Design review of the part built by this model. Coordinates are the model's own, in mm. A direction names the side the tool comes from. Coordinates: 2 decimals unless noted, no trailing zeros. Loops run counter-clockwise (first coordinate to the right, second up) from the corner with the lowest first, then second, coordinate; pieces in that order, holes last. Notation, with made-up numbers: (-5.75, 24) - (46.25, 24) arc R23 ccw to (46.25, 34) - close; hole circle Ø7 at (54.25, 34). An arc over 180 degrees is marked (long way). One line per question, with ' | ' between items.
from build123d import *

# Parameters (mm, degrees)
F0_W           = 150
F0_H           = 150
F0_R           = 30
F1_DEPTH       = 50
F2_R           = 37.5
F2_R_2         = 30
F3_DEPTH       = 40
F4_R           = 41.25
F4_R_2         = 37.5
F5_DEPTH       = 7
F7_D           = 10.2
F7_DEPTH       = 40
F7_CSINK_D     = 12
F7_CSINK_ANGLE = 90
F7_TIP         = 3.064389157
F8_R           = 15


with BuildPart() as f1:
    # F0 (on Top) → F1 (new body)
    with BuildSketch(Plane.XY):
        Rectangle(F0_W, F0_H)
        Circle(F0_R, mode=Mode.SUBTRACT)
    extrude(amount=-F1_DEPTH)

    # F2 (on face) → F3 (cut)
    with BuildSketch(Plane.XY):
        Circle(F2_R)
        Circle(F2_R_2, mode=Mode.SUBTRACT)
    extrude(amount=-F3_DEPTH, mode=Mode.SUBTRACT)

    # F4 (on face) → F5 (cut)
    with BuildSketch(Plane.XY):
        Circle(F4_R)
        Circle(F4_R_2, mode=Mode.SUBTRACT)
    extrude(amount=-F5_DEPTH, mode=Mode.SUBTRACT)

    # F7
    with Locations(Plane.XY):
        with Locations((-52.25, 52.25), (52.25, 52.25), (52.25, -52.25), (-52.25, -52.25)):
            CounterSinkHole(F7_D / 2, F7_CSINK_D / 2, depth=F7_DEPTH, counter_sink_angle=F7_CSINK_ANGLE)
            with Locations((0, 0, -(F7_DEPTH + F7_TIP / 2))):  # 118° drill point
                Cone(0, F7_D / 2, F7_TIP, mode=Mode.SUBTRACT)

    # F8
    f8_edges = [f1.edges().sort_by_distance(p)[0] for p in [
        (-75, 75, -25),
        (75, 75, -25),
        (75, -75, -25),
        (-75, -75, -25),
    ]]
    fillet(f8_edges, radius=F8_R)


solid = f1.part
Q1. For pin 1 (8 mm diameter, centred on x = 52.25, y = -52.25, fed in from +Z); pin 2 (11.5 mm diameter, centred on x = 52.25, y = 52.25, fed in from +Z), all flat-tipped, find the tip position at first contact; note any pin that passes through.
Returned:
pin 1: stops at z = -40.66 | pin 2: stops at z = -0.25
Q2. Take a section at A-A (x = 0). Give the boundary of the cut face in (y, z), plus the area to 3 significant figures.
Returned:
outline: (-75, -50) - (-30, -50) - (-30, -40) - (-37.5, -40) - (-37.5, -7) - (-41.25, -7) - (-41.25, 0) - (-75, 0) - close; (30, -50) - (75, -50) - (75, 0) - (41.25, 0) - (41.25, -7) - (37.5, -7) - (37.5, -40) - (30, -40) - close | area: 3,850 mm²
Q3. Tool access review of faces 1 (the cylindrical face through (56.009, -48.803, -20.724)), 2 (the flat face through (75, -1, -25)): name each direction out of +Z, -Z, +X, -X, +Y, -Y from which nothing blocks a thin tool from reaching the whole face with its end or side.
Returned:
face 1: +Z | face 2: +Z, -Z, +X, +Y, -Y
Q4. Draft analysis for pull direction X (two halves, no side actions). For faces 3 (the cylindrical face through (-48.491, 55.697, -20.724)), 4 (the cylindrical face through (70.49, 70.72, -25.35)), 5 (the flat face through (-75, -1, -25)), 6 (the conical face through (53.07, -52.59, -42.53)), state which applies: +X half, -X half, draft (parallel to the pull), parting line (faces both ways), or undercut.
Returned:
face 3: undercut | face 4: +X half | face 5: -X half | face 6: undercut
Q5. Take a section at C-C (z = -14). Give the boundary of the cut face in (x, y).
Returned:
outline: (-75, -60) arc R15 ccw to (-60, -75) - (60, -75) arc R15 ccw to (75, -60) - (75, 60) arc R15 ccw to (60, 75) - (-60, 75) arc R15 ccw to (-75, 60) - close; hole circle Ø10.2 at (-52.25, -52.25); hole circle Ø10.2 at (-52.25, 52.25); hole circle Ø75 at (0, 0); hole circle Ø10.2 at (52.25, -52.25); hole circle Ø10.2 at (52.25, 52.25)
Q6. Take a section at D-D (z = -45). Give the boundary of the cut face in (x, y), plus the area to 3 significant figures.
Returned:
outline: (-75, -60) arc R15 ccw to (-60, -75) - (60, -75) arc R15 ccw to (75, -60) - (75, 60) arc R15 ccw to (60, 75) - (-60, 75) arc R15 ccw to (-75, 60) - close; hole circle Ø60 at (0, 0) | area: 19,500 mm²
Q7. To check wall thickness, follow line 1 along Y through (x, z) = (52.25, -26); line 2 along Y through (x, z) = (0, -21). State the ranges of each line that lie inside material, in increasing order.
Returned:
line 1: y = -75 to -57.35, -47.15 to 47.15, 57.35 to 75 | line 2: y = -75 to -37.5, 37.5 to 75
